from build123d import *

# Parameters (mm, degrees)
SKETCH1_R          = 2.5
EXTRUDE1_DEPTH     = 100
CHAMFER1_SIZE      = 0.5
SKETCH3_W          = 19.542499602
SKETCH3_H          = 13.436538206
CUT_EXTRUDE1_DEPTH = 175


with BuildPart() as part:
    # Sketch1 → Extrude1 (new, symmetric)
    with BuildSketch(Plane.XY):
        Circle(SKETCH1_R)
    extrude(amount=EXTRUDE1_DEPTH, both=True)

    # Chamfer1
    chamfer1_edges = [part.edges().sort_by_distance(p)[0] for p in [
        (-2.5, 0, -100),
        (-2.5, 0, 100),
    ]]
    chamfer(chamfer1_edges, length=CHAMFER1_SIZE)

    # Sketch3 → Cut-Extrude1 (cut)
    with BuildSketch(Plane.XY.offset(100)):
        Rectangle(SKETCH3_W, SKETCH3_H)
    extrude(amount=-CUT_EXTRUDE1_DEPTH, mode=Mode.SUBTRACT)


solid = part.part
Check sheet for the modelled part. Datum: model origin and axes. Units: mm. Coordinates: 2 decimals unless noted, no trailing zeros. Loops run counter-clockwise (first coordinate to the right, second up) from the corner with the lowest first, then second, coordinate; pieces in that order, holes last. Notation, with made-up numbers: (-19, 61.25) -> (35, 61.25) arc R28 ccw to (35, 86.25) -> close; hole circle Ø9 at (56.25, 88). An arc over 180 degrees is marked (long way). Write item = value, one per line. Start each with the question number.
1. Depth check by flat-ended pin: P1, Ø2, axis at x = -1.5, z = -82.5, coming from the -Y side. Enter the tip coordinate at first touch or a pass-through.
2. Material ranges on line 1 (Y direction, x = 0.1, z = -81); line 2 (Y direction, x = -0.5, z = -93.75); line 3 (X direction, y = -1.75, z = -86), recorded low to high.
3. Section check A-A on z = -93. Record the cut outline in (x, y), then the cut area to 3 significant figures.
Responses:
q1.P1 = -2.45
q2.line_1 = -2.5 to 2.5
q2.line_2 = -2.45 to 2.45
q2.line_3 = -1.79 to 1.79
q3.outline = circle Ø5 at (0, 0)
q3.area = 19.6 mm2
